Autodesk Inventor part; units mm, degrees
ref_plane "YZ Plane" through (0, 0, 0) normal (1, 0, 0) x (0, 1, 0)
ref_plane "XZ Plane" through (0, 0, 0) normal (0, 1, 0) x (-1, 0, 0)
ref_plane "XY Plane" through (0, 0, 0) normal (0, 0, 1) x (1, 0, 0)
sketch "Sketch1" plane through (0, 0, 0) normal (0, 0, 1) x (1, 0, 0)
  line L0 (-17.5, 0) -> (17.5, 0) construction
  line L1 (0, -34.86) -> (0, 34.86) construction
  line L2 (-12.5, 24.9) -> (12.5, 24.9)
  line L3 (12.5, 24.9) -> (12.5, -24.9)
  line L4 (12.5, -24.9) -> (-12.5, -24.9)
  line L5 (-12.5, -24.9) -> (-12.5, 24.9)
  line L6 (-10.25, 21.4) -> (10.25, 21.4)
  line L7 (10.25, 21.4) -> (10.25, -21.4)
  line L8 (10.25, -21.4) -> (-10.25, -21.4)
  line L9 (-10.25, -21.4) -> (-10.25, 21.4)
  point P0 (0, 0)
  dimension "d0" = 20.5
  dimension "d1" = 25
  dimension "d2" = 49.8
  dimension "d3" = 42.8
extrude "Extrusion1" add sketch "Sketch1" along normal blind 3
properties part number "20_Cube_Insert_Sample_clamp"
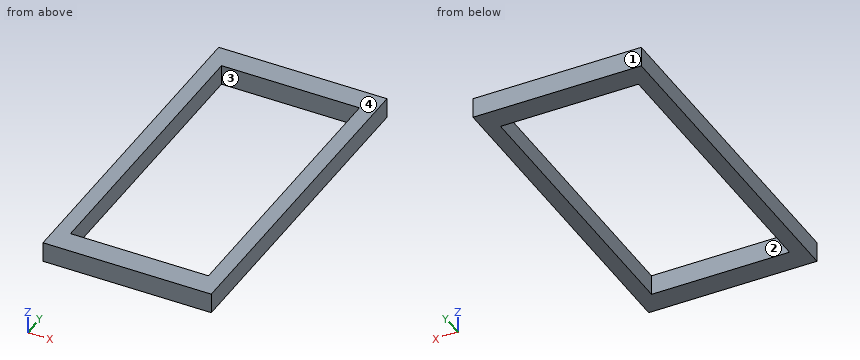
For this review, take the finished solid that the model builds, in its own axes (mm). Face numbers are marked on the shaded views. Coordinates: 2 decimals unless noted, no trailing zeros. Loops run counter-clockwise (first coordinate to the right, second up) from the corner with the lowest first, then second, coordinate; pieces in that order, holes last. Notation, with made-up numbers: (-19.75, 15.5) -> (17.25, 15.5) arc R11 cw to (17.25, 24.5) -> close; hole circle Ø7 at (-19, 62.25). An arc over 180 degrees is marked (long way). Return JSON: item names as keys, results as strings. Group by question number.
(1) Consider section C-C, the plane x = -6.5. Give the boundary of the cut face in (y, z).
(2) Consider section A-A, the plane y = 16. Give the boundary of the cut face in (x, z).
(3) Mouldability with a two-part tool opening along Y and no side actions: class the marked faces 1, 2, 3 and 4 as pulls with the +Y half, pulls with the -Y half, needs draft (parallel to the pull), parting line crosses it, or undercut.
(4) To check wall thickness, follow L1, parallel to X at y = -6, z = 0.55; L2, parallel to Y at x = -1, z = 0.75. State the ranges of each line that lie inside material, in increasing order.
(5) Consider section B-B, the plane z = 2.3. Give the boundary of the cut face in (x, y).
Results below:
{
 "1": {"outline": "(-24.9, 0) -> (-21.4, 0) -> (-21.4, 3) -> (-24.9, 3) -> close; (21.4, 0) -> (24.9, 0) -> (24.9, 3) -> (21.4, 3) -> close"},
 "2": {"outline": "(-12.5, 0) -> (-10.25, 0) -> (-10.25, 3) -> (-12.5, 3) -> close; (10.25, 0) -> (12.5, 0) -> (12.5, 3) -> (10.25, 3) -> close"},
 "3": {"face 1": "pulls with the +Y half", "face 2": "undercut", "face 3": "undercut", "face 4": "needs draft"},
 "4": {"L1": "x = -12.5 to -10.25, 10.25 to 12.5", "L2": "y = -24.9 to -21.4, 21.4 to 24.9"},
 "5": {"outline": "(-12.5, -24.9) -> (12.5, -24.9) -> (12.5, 24.9) -> (-12.5, 24.9) -> close; hole (-10.25, -21.4) -> (10.25, -21.4) -> (10.25, 21.4) -> (-10.25, 21.4) -> close"}
}
